Drawing for the job (mm, zero at the part's lowest x, y, z). Round coordinates to 2 decimals unless told otherwise and drop trailing zeros. Loops run counter-clockwise (first coordinate to the right, second up) from the corner with the lowest first, then second, coordinate; pieces in that order, holes last. Notation, with made-up numbers: M 50,31 L 55,31 A19 ccw 55,45 Z; hole C -6,2 d2. An arc over 180 degrees is marked long. Answer in a Markdown table with one row per item.
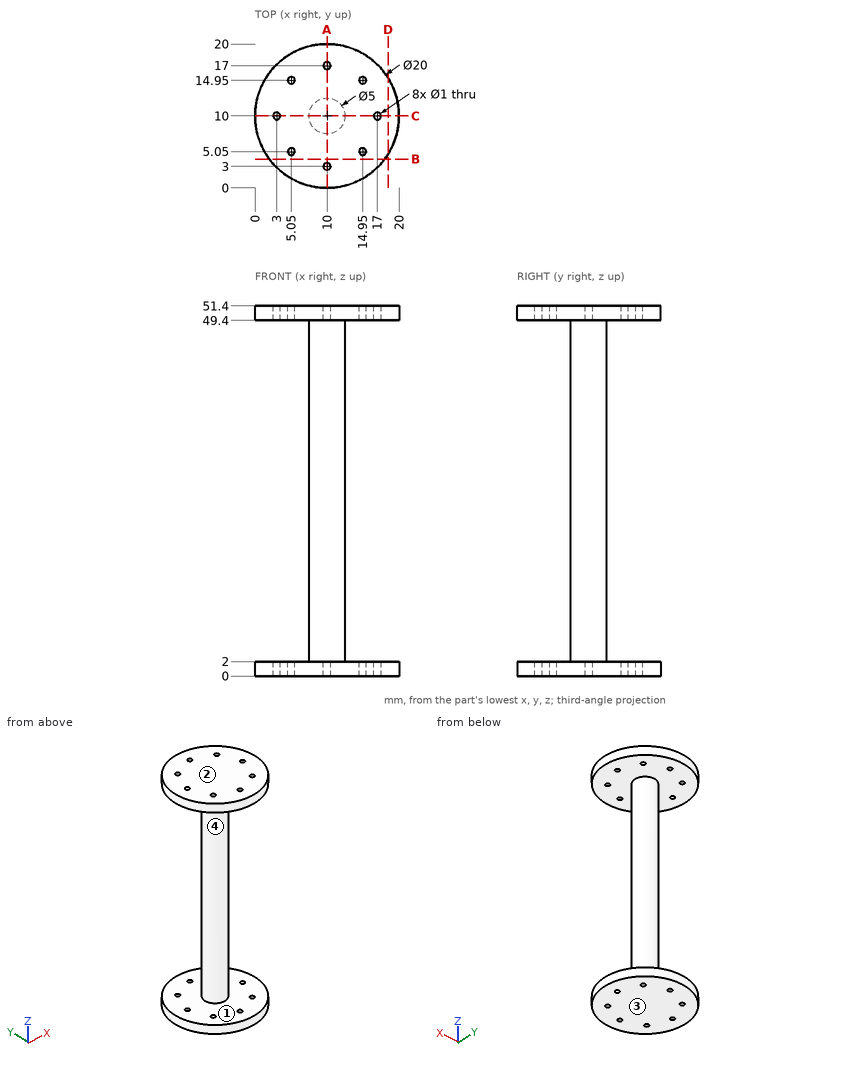
1. Pin check, flat tips, straight feed: pin 1 (4 mm diameter, centred on y = 14, z = 30.5, fed in from +X); pin 2 (10 mm diameter, centred on x = 10, z = 16, fed in from +Y); pin 3 (1.5 mm diameter, centred on x = 12.5, z = 14, fed in from -Y) (1 decimal); pin 4 (4 mm diameter, centred on x = 4, z = 41.5, fed in from -Y). Stop position of each tip, or through.
Verdict:
| item | result |
|---|---|
| pin 1 | stops at x = 11.5 |
| pin 2 | stops at y = 12.5 |
| pin 3 | stops at y = 8.2 |
| pin 4 | passes through |
2. Saw through at D-D (x = 18.5). Write the cut outline in (y, z).
Verdict:
| item | result |
|---|---|
| outline | M 4.73,0 L 15.27,0 L 15.27,2 L 4.73,2 Z; M 4.73,49.4 L 15.27,49.4 L 15.27,51.4 L 4.73,51.4 Z |
3. Saw through at A-A (x = 10). Write the cut outline in (y, z).
Verdict:
| item | result |
|---|---|
| outline | M 0,0 L 2.5,0 L 2.5,2 L 0,2 Z; M 0,49.4 L 2.5,49.4 L 2.5,51.4 L 0,51.4 Z; M 3.5,0 L 16.5,0 L 16.5,2 L 12.5,2 L 12.5,49.4 L 16.5,49.4 L 16.5,51.4 L 3.5,51.4 L 3.5,49.4 L 7.5,49.4 L 7.5,2 L 3.5,2 Z; M 17.5,0 L 20,0 L 20,2 L 17.5,2 Z; M 17.5,49.4 L 20,49.4 L 20,51.4 L 17.5,51.4 Z |
4. Mould opens along Z. For the marked faces 1, 2, 3 and 4 say: +Z half, -Z half, draft (parallel to the pull), parting line (faces both ways), or undercut.
Verdict:
| item | result |
|---|---|
| face 1 | undercut |
| face 2 | +Z half |
| face 3 | -Z half |
| face 4 | undercut |
5. Saw through at B-B (y = 4). Write the cut outline in (x, z), and give its area (3 significant figures).
Verdict:
| item | result |
|---|---|
| outline | M 2,0 L 18,0 L 18,2 L 2,2 Z; M 2,49.4 L 18,49.4 L 18,51.4 L 2,51.4 Z |
| area | 64.0 mm² |
6. Wall check: probe 1 along Y at (x, z) = (10, 49.95); probe 2 along Z at (x, y) = (17.75, 4.75); probe 3 along X at (y, z) = (3, 1.3). Give the ranges that are in metal, low to high.
Verdict:
| item | result |
|---|---|
| probe 1 | y = 0 to 2.5, 3.5 to 16.5, 17.5 to 20 |
| probe 2 | z = 0 to 2, 49.4 to 51.4 |
| probe 3 | x = 2.86 to 9.5, 10.5 to 17.14 |
